from build123d import *

# Parameters (mm, degrees)
F0_R          = 127
F1_DEPTH      = 254
F2_R          = 25.4
F3_SIZE       = 25.4
F4_R          = 44.390641743
F5_DEPTH      = 127.001
F5_DEPTH_BACK = 127.001


with BuildPart() as f1:
    # F0 (on Top) → F1 (new body)
    with BuildSketch(Plane.XY):
        Circle(F0_R)
    extrude(amount=F1_DEPTH)

    # F2
    f2_edges = [f1.edges().sort_by_distance(p)[0] for p in [
        (-127, 0, 254),
    ]]
    fillet(f2_edges, radius=F2_R)

    # F3
    f3_edges = [f1.edges().sort_by_distance(p)[0] for p in [
        (-127, 0, 0),
    ]]
    chamfer(f3_edges, length=F3_SIZE)

    # F4 (on Front) → F5 (cut, two sides)
    with BuildSketch(Plane.XZ) as f5_sk:
        with Locations((0, 125.6312429905)):
            Circle(F4_R)
    extrude(amount=-F5_DEPTH, mode=Mode.SUBTRACT)
    extrude(f5_sk.sketch, amount=F5_DEPTH_BACK, mode=Mode.SUBTRACT)


solid = f1.part
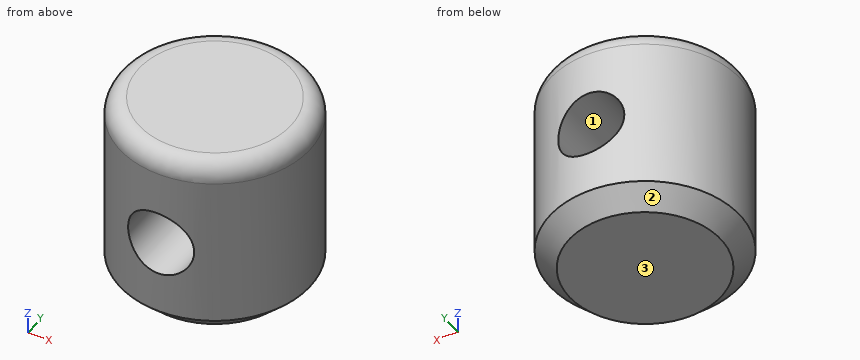
Geometry check sheet. Reference: the model listing, model coordinates, mm. Face numbers are marked on the shaded views. Coordinates: 2 decimals unless noted, no trailing zeros. Loops run counter-clockwise (first coordinate to the right, second up) from the corner with the lowest first, then second, coordinate; pieces in that order, holes last. Notation, with made-up numbers: (2, -27.75) - (51, -27.75) arc R18 ccw to (51, -20.75) - close; hole circle Ø8 at (-5.75, 33.5). An arc over 180 degrees is marked (long way). Use one line per item in the form item = value. Start each with the question number.
Item 1: Thickness scan on probe 1 along Z at (x, y) = (0, 26); probe 2 along Z at (x, y) = (29.5, -12.5); probe 3 along X at (y, z) = (23.5, 122). Record the ranges inside material, lowest first.
Item 2: Mould release check, pull along X, two halves, no side actions. Record for the marked faces 1, 2 and 3: +X half, -X half, draft (parallel to the pull), parting line (faces both ways), or undercut.
Item 3: Section check B-B, the plane y = 0. Enter the section's corners in (x, z), and give its area (3 significant figures).
Item 4: Section check A-A, the plane x = 0. Enter the section's corners in (y, z).
Item 5: Section check C-C, the plane z = 35. Enter the section's corners in (x, y), and give its area (3 significant figures).
Item 6: Gauge pin test, flat ends, axial feed: pin 1 (5 mm diameter, centred on x = -99, y = -39, fed in from +Z); pin 2 (3 mm diameter, centred on y = 88, z = 204.5, fed in from +X); pin 3 (2 mm diameter, centred on x = 39.5, y = 38, fed in from -Z); pin 4 (6 mm diameter, centred on x = 25.5, z = 40.5, fed in from +Y). Record the tip position at first contact, or that the pin passes through.
Computed:
q1.probe_1 = 0 to 81.24, 170.02 to 254
q1.probe_2 = 0 to 92.46, 158.8 to 254
q1.probe_3 = -124.81 to -44.24, 44.24 to 124.81
q2.face_1 = undercut
q2.face_2 = parting line
q2.face_3 = draft
q3.outline = (-127, 25.4) - (-101.6, 0) - (101.6, 0) - (127, 25.4) - (127, 228.6) arc R25.4 ccw to (101.6, 254) - (-101.6, 254) arc R25.4 ccw to (-127, 228.6) - close; hole circle Ø88.78 at (0, 125.63)
q3.area = 57,400 mm2
q4.outline = (-127, 25.4) - (-101.6, 0) - (101.6, 0) - (127, 25.4) - (127, 81.24) - (-127, 81.24) - close; (-127, 170.02) - (127, 170.02) - (127, 228.6) arc R25.4 ccw to (101.6, 254) - (-101.6, 254) arc R25.4 ccw to (-127, 228.6) - close
q5.outline = circle Ø254 at (0, 0)
q5.area = 50,700 mm2
q6.pin_1 = 253.9
q6.pin_2 = 92.99
q6.pin_3 = 0
q6.pin_4 = 124.99
